Verification items for the finished model (mm, model axes). Coordinates: 2 decimals unless noted, no trailing zeros. Write each loop counter-clockwise with the first axis right and the second up, starting at its lowest first coordinate (ties: lowest second). Pieces come first, ordered by that corner, then holes. Notation, with made-up numbers: M 25.25,39.25 L 44.25,39.25 A26 ccw 44.25,74.25 Z; hole C -17.75,46 d1. An arc over 180 degrees is marked long. One line per item, written item: value.
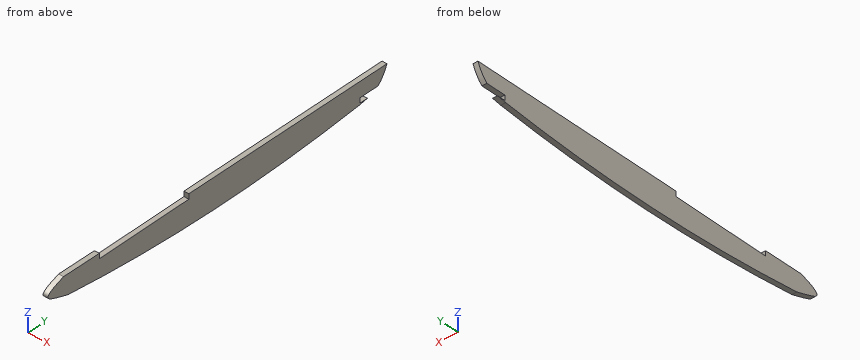
```python
from build123d import *

# Parameters (mm, degrees)
F1_DEPTH = 6.35


with BuildPart() as f1:
    # F0 (on Right) → F1 (new body)
    with BuildSketch(Plane.YZ):
        with BuildLine():
            Line((-151.8980418446, 6.0759130949), (-151.8980418446, 12.4565647503))
            Line((-151.8980418446, 12.4565647503), (-202.891856432, 12.7))
            add(Edge.make_bspline(
                [(-202.891856432, 12.7), (-215.1206120084, 8.6726070091), (-237.16462935, -1.3730042529), (-209.9079122757, -7.5103641369), (-196.4285242841, -11.9496378127)],
                knots=[0, 0, 0, 0, 0.4756763375, 1, 1, 1, 1], degree=3))
            ThreePointArc((-196.4285242841, -11.9496378127), (10.2042676339, -24.674803041), (216.9561811447, -14.0593998225))
            Line((216.9561811447, -14.0593998225), (228.6390024621, -12.1845068598))
            Line((228.6390024621, -12.1845068598), (218.3601457434, -12.1845068598))
            Line((218.3601457434, -12.1845068598), (218.3601457434, -5.8345068598))
            Line((218.3601457434, -5.8345068598), (243.7601457434, -5.8345068598))
            add(Edge.make_bspline(
                [(243.7601457434, -5.8345068598), (248.7731428179, -1.2775582425), (253.2495546938, 5.3213927641), (256.392930619, 13.4012833565)],
                knots=[19.1722123796, 19.1722123796, 19.1722123796, 19.1722123796, 38.5768547936, 38.5768547936, 38.5768547936, 38.5768547936], degree=3))
            Line((256.392930619, 13.4012833565), (-24.8988723263, 13.4012833565))
            Line((-24.8988723263, 13.4012833565), (-24.8988723263, 7.0512833565))
            Line((-24.8988723263, 7.0512833565), (-151.8980418446, 6.0759130949))
        make_face()
    extrude(amount=F1_DEPTH)


solid = f1.part
```
Item 1: Cross-section at B-B, the plane y = -48. Enter the section's corners in (x, z).
The answers:
outline: M 0,-23.45 L 6.35,-23.45 L 6.35,6.87 L 0,6.87 Z
Item 2: Cross-section at A-A, the plane y = -190. Enter the section's corners in (x, z).
The answers:
outline: M 0,-12.7 L 6.35,-12.7 L 6.35,12.64 L 0,12.64 Z
Item 3: Scan lines: line 1 (Z direction, x = 3.25, y = 230); line 2 (Z direction, x = 4.25, y = 76.5); line 3 (Y direction, x = 3.25, z = 8). Record each from-to range of solid material in increasing order.
The answers:
line 1: z = -5.83 to 13.4
line 2: z = -23.82 to 13.4
line 3: y = -215.28 to -151.9, -24.9 to 253.99
Item 4: Go/stop test with flat-tipped pins: P1, Ø1.9, axis at x = 2.5, z = 10.5, coming from the +Y side; P2, Ø1, axis at x = 1, z = -2, coming from the +Y side; P3, Ø1.9, axis at x = 2, z = -9, coming from the +Y side. Record where each tip stops, or that it passes through.
The answers:
P1: stops at y = 255.6
P2: stops at y = 247.86
P3: stops at y = 218.36
